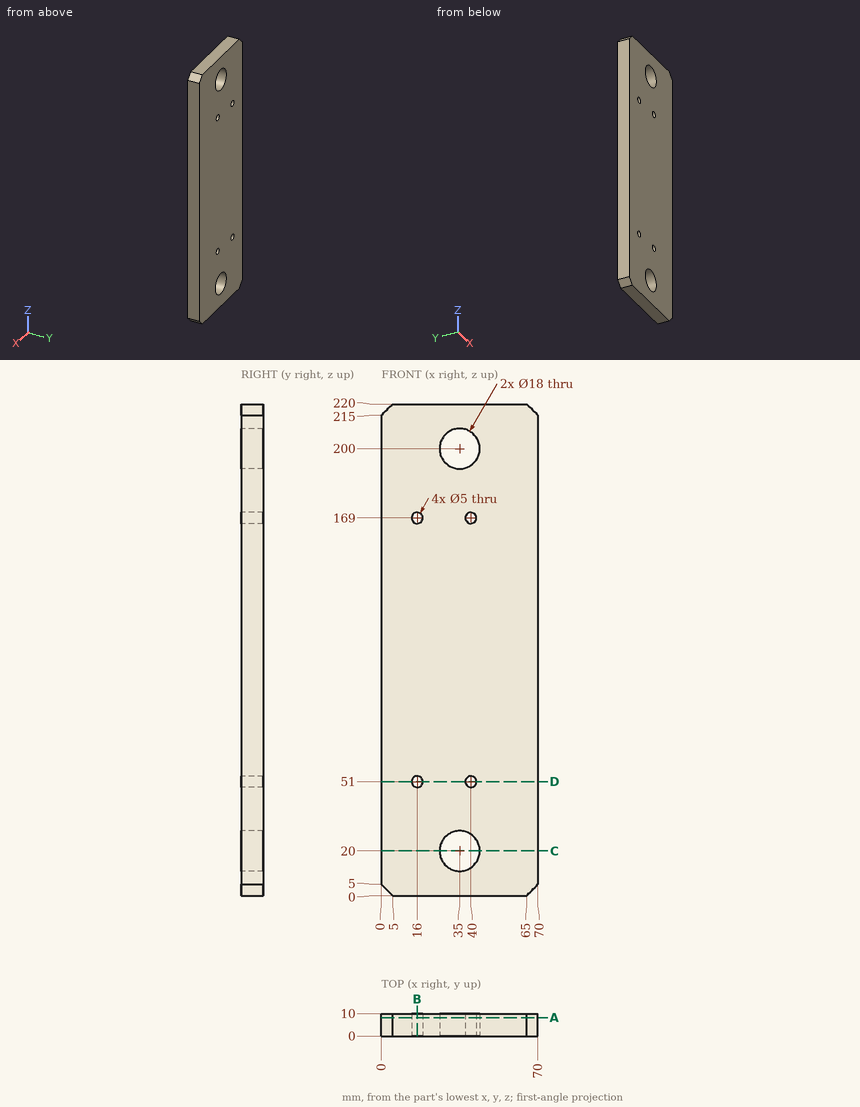
For this review, use the dimensioned drawing (mm, ordinates from the lowest corner) and the shaded views. Coordinates: 2 decimals unless noted, no trailing zeros. Write each loop counter-clockwise with the first axis right and the second up, starting at its lowest first coordinate (ties: lowest second). Pieces come first, ordered by that corner, then holes. Notation, with made-up numbers: (82, 67) - (102, 67) arc R13 ccw to (102, 87) - close; hole circle Ø10 at (-24, -12). An arc over 180 degrees is marked (long way). Answer as a JSON object with one key per item and string values. Group by question number.
1. Add section C-C (z = 20). Give the boundary of the cut face in (x, y), plus the area to 3 significant figures.
2. Add section A-A (y = 8.25). Give the boundary of the cut face in (x, z).
3. To check wall thickness, follow probe 1 along Z at (x, y) = (35, 3.5); probe 2 along X at (y, z) = (7, 53); probe 3 along Z at (x, y) = (27.5, 7.25). State the ranges of each line that lie inside material, in increasing order.
4. Add section D-D (z = 51). Give the boundary of the cut face in (x, y), plus the area to 3 significant figures.
5. Add section B-B (x = 16). Give the boundary of the cut face in (y, z).
Findings:
{
 "1": {"outline": "(0, 0) - (26, 0) - (26, 10) - (0, 10) - close; (44, 0) - (70, 0) - (70, 10) - (44, 10) - close", "area": "520 mm²"},
 "2": {"outline": "(0, 5) - (5, 0) - (65, 0) - (70, 5) - (70, 215) - (65, 220) - (5, 220) - (0, 215) - close; hole circle Ø5 at (16, 51); hole circle Ø5 at (16, 169); hole circle Ø18 at (35, 20); hole circle Ø18 at (35, 200); hole circle Ø5 at (40, 51); hole circle Ø5 at (40, 169)"},
 "3": {"probe 1": "0 to 11, 29 to 191, 209 to 220", "probe 2": "0 to 14.5, 17.5 to 38.5, 41.5 to 70", "probe 3": "0 to 15.03, 24.97 to 195.03, 204.97 to 220"},
 "4": {"outline": "(0, 0) - (13.5, 0) - (13.5, 10) - (0, 10) - close; (18.5, 0) - (37.5, 0) - (37.5, 10) - (18.5, 10) - close; (42.5, 0) - (70, 0) - (70, 10) - (42.5, 10) - close", "area": "600 mm²"},
 "5": {"outline": "(0, 0) - (10, 0) - (10, 48.5) - (0, 48.5) - close; (0, 53.5) - (10, 53.5) - (10, 166.5) - (0, 166.5) - close; (0, 171.5) - (10, 171.5) - (10, 220) - (0, 220) - close"}
}
